Part model, mm, in its own coordinate system. A direction names the side the tool comes from. Give positions to 0.01 mm unless a question says otherwise; leave off trailing zeros. Write each loop counter-clockwise with the first axis right and the second up, starting at its lowest first coordinate (ties: lowest second). Pieces come first, ordered by that corner, then holes. Notation, with made-up numbers: (11.25, 60.5) - (60.25, 60.5) arc R25 ccw to (60.25, 73.5) - close; hole circle Ø5 at (30.25, 30). An arc over 180 degrees is marked (long way). Answer as a JSON object with one key per item and string values. Group by question number.
```python
from build123d import *

# Parameters (mm, degrees)
BOX162_W     = 9
BOX162_H     = 2
BOX162_DEPTH = 2
BOX160_W     = 2
BOX160_H     = 10.25
BOX160_DEPTH = 2


with BuildPart() as cube151:
    # Box162 → Box162 (new body)
    with BuildSketch(Plane(origin=(43.5, 28.25, 2), x_dir=(1, 0, 0), z_dir=(0, 0, 1))):
        with Locations((4.5, 1)):
            Rectangle(BOX162_W, BOX162_H)
    extrude(amount=BOX162_DEPTH)


with BuildPart() as fusion050:
    # Box160 → Box160 (new body)
    with BuildSketch(Plane(origin=(41.5, 20, 2), x_dir=(1, 0, 0), z_dir=(0, 0, 1))):
        with Locations((1, 5.125)):
            Rectangle(BOX160_W, BOX160_H)
    extrude(amount=BOX160_DEPTH)

    # Fusion050: union Cube151
    add(cube151.part)


solid = fusion050.part
```
1) Which spindle directions (+Z, -Z, +X, -X, +Y, -Y) get a long thin tool onto all of the face, cutting with end or side? Do faces 1 (the flat face through (47, 30.25, 3)), 2 (the flat face through (48, 28.25, 3)). Say none if no direction does.
2) Drop a flat-ended pin along its axis: P1, Ø0.6, axis at y = 26, z = 3.5, coming from the +X side. Give the stop position or say it passes through.
3) Probe line 1 (X direction, y = 24.5, z = 2.45); line 2 (Y direction, x = 44.25, z = 2.9). List the from-to ranges inside material, lowest first.
4) Band-saw the part on C-C (x = 51). List the corners of the cut face in (y, z), plus the area to 3 significant figures.
5) Band-saw the part on A-A (z = 3.1). List the corners of the cut face in (x, y).
6) Band-saw the part on B-B (y = 27). List the corners of the cut face in (x, z), plus the area to 3 significant figures.
Verdict:
{
 "1": {"face 1": "+Z, -Z, +X, -X, +Y", "face 2": "+Z, -Z, +X, -Y"},
 "2": {"P1": "x = 43.5"},
 "3": {"line 1": "41.5 to 43.5", "line 2": "28.25 to 30.25"},
 "4": {"outline": "(28.25, 2) - (30.25, 2) - (30.25, 4) - (28.25, 4) - close", "area": "4.00 mm2"},
 "5": {"outline": "(41.5, 20) - (43.5, 20) - (43.5, 28.25) - (52.5, 28.25) - (52.5, 30.25) - (41.5, 30.25) - close"},
 "6": {"outline": "(41.5, 2) - (43.5, 2) - (43.5, 4) - (41.5, 4) - close", "area": "4.00 mm2"}
}
